from build123d import *

# Parameters (mm, degrees)
SALIENTE_EXTRUIR1_DEPTH = 10
CROQUIS2_R              = 1.5
CROQUIS2_W              = 55
CROQUIS2_H              = 3
CORTAR_EXTRUIR1_DEPTH   = 10
CROQUIS3_W              = 15
CROQUIS3_H              = 2.5
CORTAR_EXTRUIR2_DEPTH   = 10
CROQUIS4_R              = 1.5
CORTAR_EXTRUIR3_DEPTH   = 10
CORTAR_EXTRUIR5_DEPTH   = 10
CROQUIS9_R              = 2
SALIENTE_EXTRUIR2_DEPTH = 2.5
CROQUIS10_W             = 70
CROQUIS10_H             = 16.144583998
CORTAR_EXTRUIR6_DEPTH   = 10


with BuildPart() as part:
    # Croquis1 → Saliente-Extruir1 (new body)
    with BuildSketch(Plane.XY):
        Polygon((0, 0), (105, 0), (105, 2.5), (105, 7.5), (105, 10), (0, 10), (0, 7.5), (15, 7.5), (15, 2.5), (0, 2.5), align=None)
    extrude(amount=SALIENTE_EXTRUIR1_DEPTH)

    # Croquis2 → Cortar-Extruir1 (cut)
    with BuildSketch(Plane(origin=(0, 10, 0), x_dir=(1, 0, 0), z_dir=(0, 1, 0))):
        with Locations(Location((5, -5, 0), (0, 0, 270))):
            Circle(CROQUIS2_R)
        with BuildLine():
            Line((-4.031911586, 0), (5, 0))
            ThreePointArc((5, 0), (0, -5), (5, -10))
            Line((5, -10), (-4.031911586, -10))
            Line((-4.031911586, -10), (-4.031911586, 0))
        make_face()
        with Locations((50, -5)):
            Rectangle(CROQUIS2_W, CROQUIS2_H)
    extrude(amount=-CORTAR_EXTRUIR1_DEPTH, mode=Mode.SUBTRACT)

    # Croquis3 → Cortar-Extruir2 (cut)
    with BuildSketch(Plane(origin=(0, 10, 0), x_dir=(1, 0, 0), z_dir=(0, 1, 0))):
        with Locations((97.5, -1.25)):
            Rectangle(CROQUIS3_W, CROQUIS3_H)
        with Locations((97.5, -8.75)):
            Rectangle(CROQUIS3_W, CROQUIS3_H)
    extrude(amount=-CORTAR_EXTRUIR2_DEPTH, mode=Mode.SUBTRACT)

    # Croquis4 → Cortar-Extruir3 (cut)
    with BuildSketch(Plane.XY.offset(7.5)):
        with Locations((100, 5)):
            Circle(CROQUIS4_R)
        with BuildLine():
            Line((100, 10), (171.112400038, 10))
            Line((171.112400038, 10), (171.112400038, 0))
            Line((171.112400038, 0), (100, 0))
            ThreePointArc((100, 0), (105, 5), (100, 10))
        make_face()
    extrude(amount=-CORTAR_EXTRUIR3_DEPTH, mode=Mode.SUBTRACT)

    # Croquis8 → Cortar-Extruir5 (cut)
    with BuildSketch(Plane.XY.offset(7.5)):
        with BuildLine():
            Line((90, 0), (100, 0))
            ThreePointArc((100, 0), (105, 5), (100, 10))
            Line((100, 10), (90, 10))
            Line((90, 10), (90, 0))
        make_face()
    extrude(amount=-CORTAR_EXTRUIR5_DEPTH, mode=Mode.SUBTRACT)

    # Croquis9 → Saliente-Extruir2 (add, symmetric)
    with BuildSketch(Plane(origin=(0, 5, 0), x_dir=(-1, 0, 0), z_dir=(0, -1, 0))):
        with BuildLine():
            Line((-90, -10), (-95, -10))
            ThreePointArc((-95, -10), (-100, -5), (-95, 0))
            Line((-95, 0), (-90, 0))
            Line((-90, 0), (-90, -10))
        make_face()
        with Locations(Location((-95, -5, 0), (0, 0, 90))):
            Circle(CROQUIS9_R, mode=Mode.SUBTRACT)
    extrude(amount=SALIENTE_EXTRUIR2_DEPTH, both=True)

    # Croquis10 → Cortar-Extruir6 (cut)
    with BuildSketch(Plane(origin=(0, 0, 0), x_dir=(-1, 0, 0), z_dir=(0, 0, -1))):
        with Locations((-55, 15.572291999)):
            Rectangle(CROQUIS10_W, CROQUIS10_H)
        with Locations((-55, -5.572291999)):
            Rectangle(CROQUIS10_W, CROQUIS10_H)
    extrude(amount=-CORTAR_EXTRUIR6_DEPTH, mode=Mode.SUBTRACT)


solid = part.part
Geometry: final body of the model. Coordinates: model frame, mm. A direction names the side the tool comes from. Give positions to 0.01 mm unless a question says otherwise; leave off trailing zeros. Loops run counter-clockwise (first coordinate to the right, second up) from the corner with the lowest first, then second, coordinate; pieces in that order, holes last. Notation, with made-up numbers: M 84,-37 L 123,-37 A13 ccw 123,-19 Z; hole C 26.25,41.5 d1. An arc over 180 degrees is marked long. Put each result on its own line as item: value.
1) Mould query, pull axis X, two halves, no side actions, for faces 1 (the cylindrical face through (0, 1, 5)), 2 (the cylindrical face through (4.425, 1.268, 6.386)), 3 (the flat face through (8, 2.5, 5)). Classes: released by +X, released by -X, zero draft, split by the parting line, or undercut.
Computed values:
face 1: released by -X
face 2: undercut
face 3: zero draft
2) First-contact query: P1, Ø2.5, axis at x = 5, z = 5, coming from the +Y side; P2, Ø5, axis at y = 4.5, z = 2.5, coming from the -X side; P3, Ø1.5, axis at y = 7, z = 6.5, coming from the +X side; P4, Ø4, axis at y = 6, z = 8.5, coming from the -X side. Flat tips, straight axial feed; report the tip coordinate or a pass-through.
Computed values:
P1: passes through
P2: stops at x = 0.1
P3: stops at x = 99.94
P4: stops at x = 0.5
3) Cut plane D-D, the plane y = 9. Return the cut outline in (x, z), plus the area to 3 significant figures.
Computed values:
outline: M 5,0 L 20,0 L 20,10 L 5,10 A5 ccw Z; hole C 5,5 d3
area: 182 mm^2
4) Reachability of faces 4 (the flat face through (50, 5, 6.5)), 5 (the flat face through (7, 7.5, 5)), 6 (the flat face through (59, 2.5, 3)), 7 (the flat face through (10, 0, 5)), 8 (the flat face through (61, 7.5, 3)) from +Z, -Z, +X, -X, +Y, -Y: full face, straight path, thin tool, end or side. Return the list, or none.
Computed values:
face 4: +Y, -Y
face 5: +Z, -Z, -X
face 6: +Z, -Z, +X, -Y
face 7: +Z, -Z, +X, -X, -Y
face 8: +Z, -Z, +X, +Y
5) Material intervals for L1, parallel to X at y = 6.45, z = 5; L2, parallel to Z at x = 30.5, y = 3.25; L3, parallel to X at y = 9.3, z = 5, sorted ascending. Write a range as from..to.
Computed values:
L1: x = 15..22.5, 77.5..93, 97..100
L2: z = 0..3.5, 6.5..10
L3: x = 0..3.5, 6.5..20
6) Cut plane C-C, the plane y = 4.5. Return the cut outline in (x, z), plus the area to 3 significant figures.
Computed values:
outline: M 15,0 L 95,0 A5 ccw 95,10 L 15,10 Z; hole M 22.5,3.5 L 77.5,3.5 L 77.5,6.5 L 22.5,6.5 Z; hole C 95,5 d4
area: 662 mm^2
7) Cut plane B-B, the plane z = 5. Return the cut outline in (x, y), plus the area to 3 significant figures.
Computed values:
outline: M 0,0 L 3.5,0 L 3.5,2.5 L 0,2.5 Z; M 0,7.5 L 3.5,7.5 L 3.5,10 L 0,10 Z; M 6.5,0 L 20,0 L 20,2.5 L 22.5,2.5 L 22.5,7.5 L 20,7.5 L 20,10 L 6.5,10 L 6.5,7.5 L 15,7.5 L 15,2.5 L 6.5,2.5 Z; M 77.5,2.5 L 93,2.5 L 93,7.5 L 77.5,7.5 Z; M 97,2.5 L 100,2.5 L 100,7.5 L 97,7.5 Z
area: 215 mm^2
8) Cut plane A-A, the plane x = 29. Return the cut outline in (y, z).
Computed values:
outline: M 2.5,0 L 7.5,0 L 7.5,3.5 L 2.5,3.5 Z; M 2.5,6.5 L 7.5,6.5 L 7.5,10 L 2.5,10 Z
